Input: part model. Units: mm. Frame: model coordinates. Give positions to 0.01 mm unless a question says otherwise; leave off trailing zeros. Order: outer loops, then holes, each group sorted by start corner. A loop starts at its lowest first (then second) coordinate and runs counter-clockwise, first axis right, second up. Notation, with made-up numbers: M 38,27.25 L 48,27.25 A9 cw 48,34.25 Z; hole C 55,73 d6. An arc over 180 degrees is marked long. Use a Markdown table: item, result.
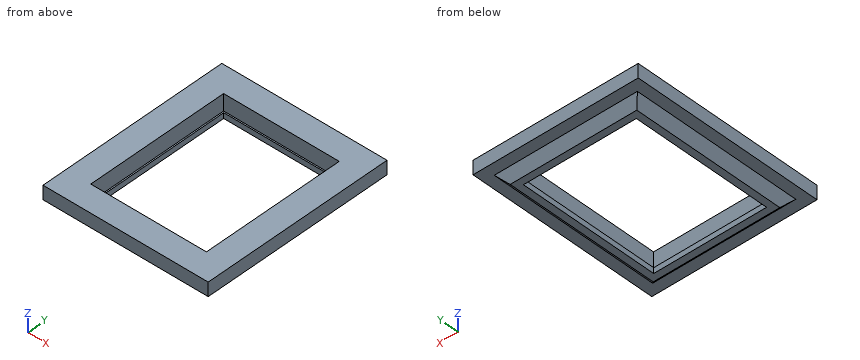
from build123d import *

# Parameters (mm, degrees)
EXTRUDE_1_DEPTH      = 6
EXTRUDE_1_DEPTH_BACK = 2
SKETCH_1_W           = 60
SKETCH_1_H           = 70
SKETCH_1_W_2         = 41
SKETCH_1_H_2         = 51
SKETCH_2_W           = 42
SKETCH_2_H           = 52
CUT_EXTRUDE_2_DEPTH  = 47.486557197
SKETCH_3_W           = 4
SKETCH_3_H           = 3
CHAMFER_2_SIZE       = 3


with BuildPart() as part:
    # Эскиз1 → Бобышка-Вытянуть1 (new, two sides: drawn at the far end of the back side and taken through both)
    with BuildSketch(Plane.XY.offset(-EXTRUDE_1_DEPTH_BACK)):
        Rectangle(SKETCH_1_W, SKETCH_1_H)
        Rectangle(SKETCH_1_W_2, SKETCH_1_H_2, mode=Mode.SUBTRACT)
    extrude(amount=EXTRUDE_1_DEPTH + EXTRUDE_1_DEPTH_BACK)

    # Эскиз2 → Вырез-Вытянуть2 (cut, through all)
    with BuildSketch(Plane(origin=(0, 0, 0), x_dir=(-1, 0, 0), z_dir=(0, 0, -1))):
        Rectangle(SKETCH_2_W, SKETCH_2_H)
    extrude(amount=-CUT_EXTRUDE_2_DEPTH, mode=Mode.SUBTRACT)

    # Вырез-По траектории1: sweep along a path in Эскиз4
    with BuildLine(Plane(origin=(0, 0, -2), x_dir=(-1, 0, 0), z_dir=(0, 0, -1))) as sweep_1_path:
        Line((-30, 35), (-30, -35))
        Line((-30, -35), (30, -35))
        Line((30, -35), (30, 35))
        Line((30, 35), (-30, 35))
    # Эскиз3 → Вырез-По траектории1 (sweep, cut)
    with BuildSketch(Plane(origin=(0, -35, 0), x_dir=(-1, 0, 0), z_dir=(0, -1, 0))):
        with Locations((-28, 0.5)):
            Rectangle(SKETCH_3_W, SKETCH_3_H)
    sweep(path=sweep_1_path.line, transition=Transition.RIGHT, mode=Mode.SUBTRACT)

    # Фаска2
    chamfer_2_edges = [part.edges().sort_by_distance(p)[0] for p in [
        (26, 0, -2),
        (0, 31, -2),
        (-26, 0, -2),
        (0, -31, -2),
    ]]
    chamfer(chamfer_2_edges, length=CHAMFER_2_SIZE - 0.0001)  # a hair under: the kernel refuses the full size


solid = part.part
1) Material intervals for line 1 (X direction, y = 17, z = 2.75); line 2 (Y direction, x = 10, z = 4.75); line 3 (Z direction, x = -26, y = 19), sorted ascending. Write a range as from..to.
Response values:
| item | result |
|---|---|
| line 1 | x = -30..-21, 21..30 |
| line 2 | y = -35..-26, 26..35 |
| line 3 | z = 1..6 |
2) First-contact query: pin 1 Ø2 at (x, z) = (1.5, -1) entering from +Y; pin 2 Ø3 at (x, y) = (18, -15) entering from -Z; pin 3 Ø2 at (y, z) = (0.5, -1.5) entering from -X; pin 4 Ø1.6 at (x, z) = (-9.5, -1.5) entering from -Y. Flat tips, straight axial feed; report the tip coordinate or a pass-through.
Response values:
| item | result |
|---|---|
| pin 1 | stops at y = 30 |
| pin 2 | passes through |
| pin 3 | stops at x = -24.5 |
| pin 4 | stops at y = -29.3 |
3) Cut plane C-C on z = 4.25. Return loops of the section in (x, y), and give its area (3 significant figures).
Response values:
| item | result |
|---|---|
| outline | M -30,-35 L 30,-35 L 30,35 L -30,35 Z; hole M -21,-26 L 21,-26 L 21,26 L -21,26 Z |
| area | 2,020 mm² |
